Part print with two shaded views. Sizes in mm from the minimum x, y, z corner. A direction names the side the tool comes from. Round coordinates to 2 decimals unless told otherwise and drop trailing zeros. Write each loop counter-clockwise with the first axis right and the second up, starting at its lowest first coordinate (ties: lowest second). Pieces come first, ordered by that corner, then holes.
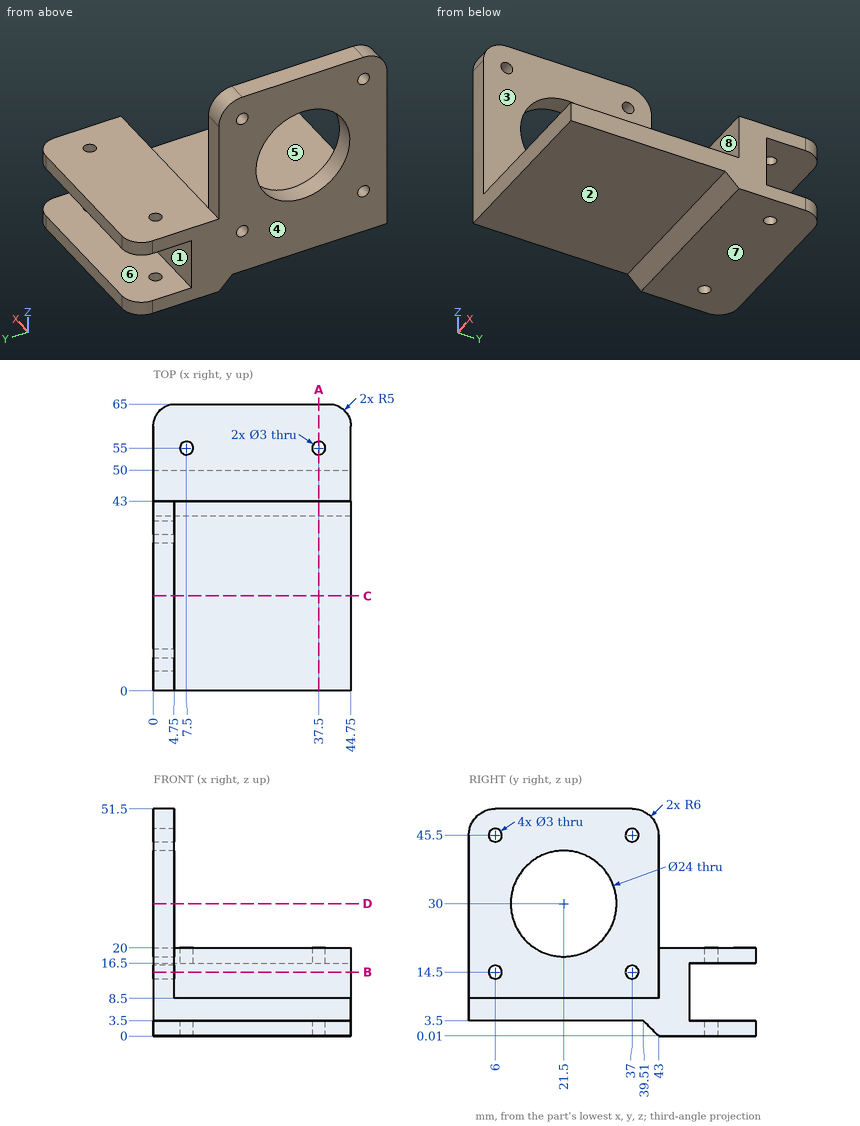
Q1. Drop flat-ended pins along their axis: pin 1 (6 mm diameter, centred on x = 31.5, z = 17, fed in from -Y); pin 2 (12 mm diameter, centred on x = 24.5, y = 60.5, fed in from +Z); pin 3 (3 mm diameter, centred on y = 7, z = 12.5, fed in from +X). Give the stop position or say it passes through.
Values follow:
pin 1: stops at y = 43
pin 2: stops at z = 20
pin 3: stops at x = 4.75
Q2. Cut at C-C on y = 21.5. Write the cut outline in (x, z), plus the area to 3 significant figures.
Values follow:
outline: (0, 3.5) - (44.75, 3.5) - (44.75, 8.5) - (4.75, 8.5) - (4.75, 18) - (0, 18) - close; (0, 42) - (4.75, 42) - (4.75, 51.5) - (0, 51.5) - close
area: 314 mm2
Q3. Mould opens along Z. For the marked faces 5, 6, 7 and 8 say: +Z half, -Z half, draft (parallel to the pull), parting line (faces both ways), or undercut.
Values follow:
face 5: +Z half
face 6: undercut
face 7: -Z half
face 8: draft
Q4. Wall check: L1, parallel to Z at x = 2.9, y = 6; L2, parallel to Y at x = 1.9, z = 45.5; L3, parallel to Y at x = 3.75, z = 14.5. Give the ranges that are in metal, low to high.
Values follow:
L1: z = 3.5 to 13, 16 to 44, 47 to 51.5
L2: y = 0 to 4.5, 7.5 to 35.5, 38.5 to 43
L3: y = 0 to 4.5, 7.5 to 35.5, 38.5 to 50
Q5. Cut at B-B on z = 14.5. Write the cut outline in (x, y), plus the area to 3 significant figures.
Values follow:
outline: (0, 0) - (4.75, 0) - (4.75, 4.5) - (0, 4.5) - close; (0, 7.5) - (4.75, 7.5) - (4.75, 35.5) - (0, 35.5) - close; (0, 38.5) - (4.75, 38.5) - (4.75, 43) - (44.75, 43) - (44.75, 50) - (0, 50) - close
area: 489 mm2
Q6. Cut at A-A on x = 37.5. State how many separate pieces and enclosed holes the cut face has, plus the area to 3 significant figures.
Values follow:
separate pieces: 3
enclosed holes: 0
area: 445 mm2
Q7. Which spindle directions (+Z, -Z, +X, -X, +Y, -Y) get a long thin tool onto all of the face, cutting with end or side? Do the marked faces 1, 2, 3 and 4. Say none if no direction does.
Values follow:
face 1: +X, -X, +Y
face 2: -Z, +X, -X, -Y
face 3: +Z, +X, -Y
face 4: +Z, -Z, -X, +Y, -Y
Q8. Cut at D-D on z = 30. Write the cut outline in (x, y), plus the area to 4 significant figures.
Values follow:
outline: (0, 0) - (4.75, 0) - (4.75, 9.5) - (0, 9.5) - close; (0, 33.5) - (4.75, 33.5) - (4.75, 43) - (0, 43) - close
area: 90.25 mm2
